```python
from build123d import *

# Parameters (mm, degrees)
CUT_EXTRUDE1_DEPTH = 1
FILLET1_R          = 1.5
CHAMFER1_SIZE      = 0.5


with BuildPart() as part:
    # Sketch1 → Revolve1 (revolve)
    with BuildSketch(Plane(origin=(0, 0, 0), x_dir=(1, 0, 0), z_dir=(0, 1, 0))):
        Polygon((0, 0), (-8, -9.8e-16), (-8, -1.500000000000001), (1e-17, -1.5), align=None)
        Polygon((1e-17, 1.3999999999999995), (1e-17, 0), (1e-17, -1.5), (2, -1.5), (2, 1.3999999999999995), align=None)
    revolve(axis=Axis((1e-17, 0, 1.5), (-1, 0, 1.4e-16)))

    # Sketch3 → Cut-Extrude1 (cut)
    with BuildSketch(Plane(origin=(2, 0, -2.7e-16), x_dir=(-1.3e-16, 0, -1), z_dir=(1, 0, -1.3e-16))):
        Polygon((-2.2216878364870323, -1.2500000000000002), (-0.7783121635129678, -1.2500000000000002), (-0.05662432702593554, 0), (-0.7783121635129678, 1.2500000000000002), (-2.2216878364870323, 1.2500000000000004), (-2.9433756729740645, 0), align=None)
    extrude(amount=-CUT_EXTRUDE1_DEPTH, mode=Mode.SUBTRACT)

    # Fillet1
    fillet1_edges = [part.edges().sort_by_distance(p)[0] for p in [
        (2.000000000000001, -3.6e-16, 4.3999999999999995),
    ]]
    fillet(fillet1_edges, radius=FILLET1_R - 0.0001)  # a hair under: the kernel refuses the full size

    # Chamfer1
    chamfer1_edges = [part.edges().sort_by_distance(p)[0] for p in [
        (-8, -1.8e-16, 3.0000000000000013),
    ]]
    chamfer(chamfer1_edges, length=CHAMFER1_SIZE)


solid = part.part
```
Work out the finished part from the listing and answer in its coordinate system (mm). A direction names the side the tool comes from. Round coordinates to 2 decimals unless told otherwise and drop trailing zeros. Write each loop counter-clockwise with the first axis right and the second up, starting at its lowest first coordinate (ties: lowest second). Pieces come first, ordered by that corner, then holes. Notation, with made-up numbers: (74, 71) - (96, 71) arc R23 ccw to (96, 87) - close; hole circle Ø6 at (51.25, 44.5). An arc over 180 degrees is marked (long way). Return JSON: item names as keys, results as strings. Group by question number.
Q1. For faces 5 (the flat face through (0, 1, 0)), 6 (the cylindrical face through (0.247, -2.875, 1.878)), 7 (the flat face through (1.51, 0.63, 2.58)), determine the directions among +Z, -Z, +X, -X, +Y, -Y from which every point of the face is accessible in a straight line to the end or side of a thin tool.
Q2. The part is cut by section A-A on x = -1. Write down the section's boundary in (y, z), then the cut area to 3 significant figures.
Q3. The mould has two halves that part along Z. Classify faces 1 (the flat face through (-8, 0, 2)), 2 (the cylindrical face through (-4, 0, 3)), 3 (the flat face through (1.5, -1.25, 1.5)), 4 (the flat face through (1.507, 0.616, 0.412)): released by +Z, released by -Z, zero draft, split by the parting line, or undercut.
Q4. Find the intervals of material crossed by L1, parallel to Y at x = -1, z = 1.4; L2, parallel to X at y = 1.2, z = 2.85; L3, parallel to X at y = 0.85, z = -0.8, in increasing order.
Q5. Each of these flat-tipped pins is pushed along its axis until it touches: pin 1 Ø1 at (y, z) = (0, 1) entering from +X; pin 2 Ø1 at (y, z) = (-1, 0) entering from -X; pin 3 Ø1.1 at (x, z) = (1.5, 1.5) entering from +Y. Where does it stop, or does it pass through?
Solved:
{
 "1": {"face 5": "-X", "face 6": "+X, -X", "face 7": "+X"},
 "2": {"outline": "circle Ø3 at (0, 1.5)", "area": "7.07 mm²"},
 "3": {"face 1": "zero draft", "face 2": "split by the parting line", "face 3": "undercut", "face 4": "undercut"},
 "4": {"L1": "-1.5 to 1.5", "L2": "0 to 1.94", "L3": "0 to 1.57"},
 "5": {"pin 1": "x = 1", "pin 2": "x = -7.7", "pin 3": "y = 2.83"}
}
